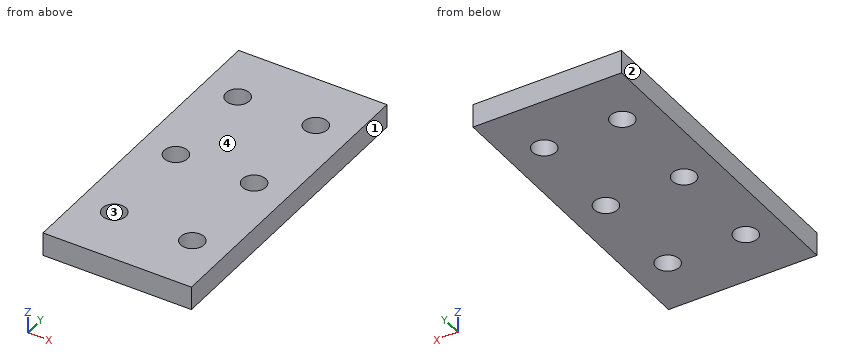
from build123d import *

# Parameters (mm, degrees)
SKETCH12_W          = 19
SKETCH12_H          = 40
SKETCH12_R          = 1.5
BOSS_EXTRUDE6_DEPTH = 3


with BuildPart() as part:
    # Sketch12 → Boss-Extrude6 (new body)
    with BuildSketch(Plane.XY):
        with Locations((-9.5, 0)):
            Rectangle(SKETCH12_W, SKETCH12_H)
        with Locations((-4.5, 0)):
            Circle(SKETCH12_R, mode=Mode.SUBTRACT)
        with Locations((-4.5, -12.625)):
            Circle(SKETCH12_R, mode=Mode.SUBTRACT)
        with Locations((-14.5, -12.625)):
            Circle(SKETCH12_R, mode=Mode.SUBTRACT)
        with Locations(Location((-4.5, 12.625, 0), (0, 0, 180))):
            Circle(SKETCH12_R, mode=Mode.SUBTRACT)
        with Locations(Location((-14.5, 12.625, 0), (0, 0, 180))):
            Circle(SKETCH12_R, mode=Mode.SUBTRACT)
        with Locations((-14.5, 0)):
            Circle(SKETCH12_R, mode=Mode.SUBTRACT)
    extrude(amount=BOSS_EXTRUDE6_DEPTH)


solid = part.part
Geometry: final body of the model. Coordinates: model frame, mm. Face numbers are marked on the shaded views. Round coordinates to 2 decimals unless told otherwise and drop trailing zeros. Order: outer loops, then holes, each group sorted by start corner. A loop starts at its lowest first (then second) coordinate and runs counter-clockwise, first axis right, second up.
Q1. Section D-D, the plane y = -13.5. Output: boundary loops of the cut face in (x, z), and give its area (3 significant figures).
Result sheet:
outline: (-19, 0) - (-15.72, 0) - (-15.72, 3) - (-19, 3) - close; (-13.28, 0) - (-5.72, 0) - (-5.72, 3) - (-13.28, 3) - close; (-3.28, 0) - (0, 0) - (0, 3) - (-3.28, 3) - close
area: 42.4 mm2
Q2. Section C-C, the plane z = 1.25. Output: boundary loops of the cut face in (x, y) (3 decimals), and give its area (3 significant figures).
Result sheet:
outline: (-19, -20) - (0, -20) - (0, 20) - (-19, 20) - close; hole circle Ø3 at (-14.5, -12.625); hole circle Ø3 at (-14.5, 0); hole circle Ø3 at (-14.5, 12.625); hole circle Ø3 at (-4.5, -12.625); hole circle Ø3 at (-4.5, 0); hole circle Ø3 at (-4.5, 12.625)
area: 718 mm2
Q3. Mould query, pull axis X, two halves, no side actions, for the marked faces 1, 2, 3 and 4. Classes: released by +X, released by -X, zero draft, split by the parting line, or undercut.
Result sheet:
face 1: released by +X
face 2: released by -X
face 3: undercut
face 4: zero draft
Q4. Pin query (flat end, axial travel): pin 1 (3.5 mm diameter, centred on x = -14.5, y = 0, fed in from -Z). Return the tip coordinate at first contact, or that it passes through.
Result sheet:
pin 1: stops at z = 0
Q5. Section A-A, the plane x = -14.5. Output: boundary loops of the cut face in (y, z) (3 decimals).
Result sheet:
outline: (-20, 0) - (-14.125, 0) - (-14.125, 3) - (-20, 3) - close; (-11.125, 0) - (-1.5, 0) - (-1.5, 3) - (-11.125, 3) - close; (1.5, 0) - (11.125, 0) - (11.125, 3) - (1.5, 3) - close; (14.125, 0) - (20, 0) - (20, 3) - (14.125, 3) - close
Q6. Section B-B, the plane y = 0. Output: boundary loops of the cut face in (x, z), and give its area (3 significant figures).
Result sheet:
outline: (-19, 0) - (-16, 0) - (-16, 3) - (-19, 3) - close; (-13, 0) - (-6, 0) - (-6, 3) - (-13, 3) - close; (-3, 0) - (0, 0) - (0, 3) - (-3, 3) - close
area: 39.0 mm2
Q7. Material intervals for probe 1 along Y at (x, z) = (-14.5, 2) (3 decimals); probe 2 along Y at (x, z) = (-13.25, 0.7); probe 3 along X at (y, z) = (12, 2.1), sorted ascending.
Result sheet:
probe 1: y = -20 to -14.125, -11.125 to -1.5, 1.5 to 11.125, 14.125 to 20
probe 2: y = -20 to -13.45, -11.8 to -0.83, 0.83 to 11.8, 13.45 to 20
probe 3: x = -19 to -15.86, -13.14 to -5.86, -3.14 to 0
